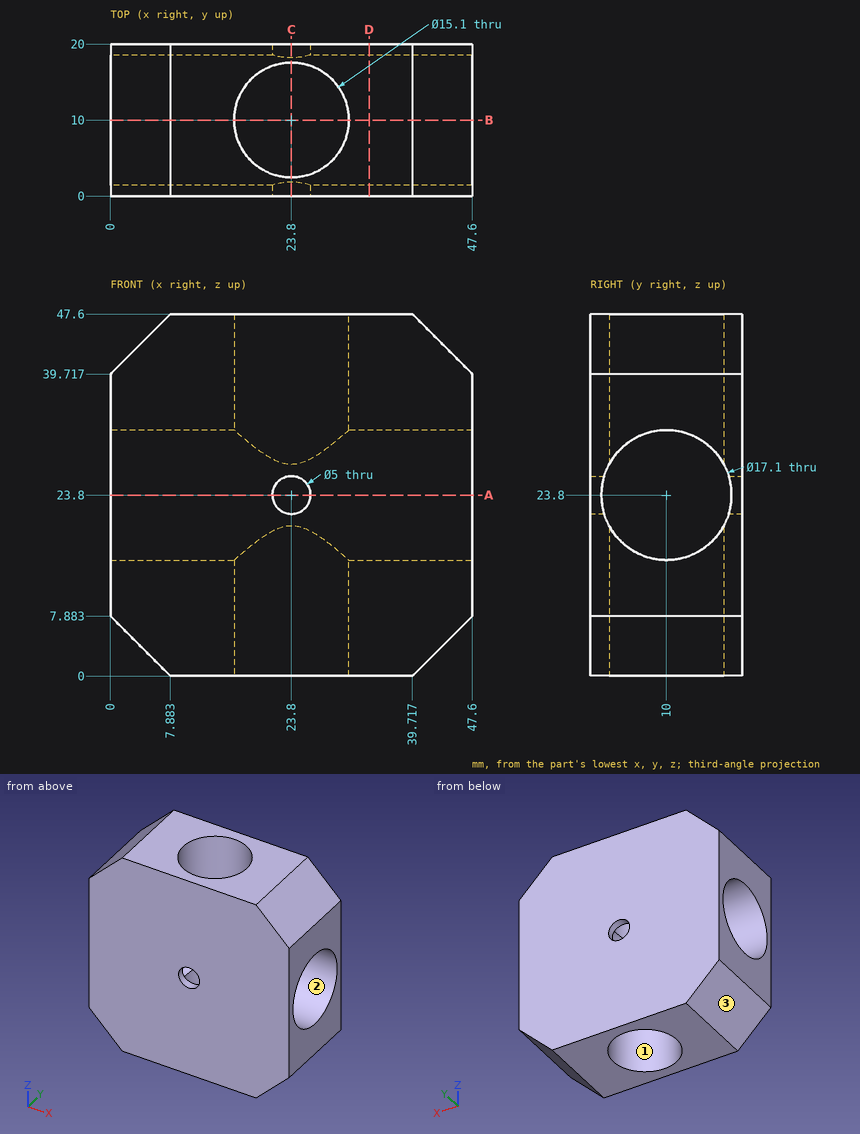
Drawing for the job (mm, zero at the part's lowest x, y, z). Round coordinates to 2 decimals unless told otherwise and drop trailing zeros. Write each loop counter-clockwise with the first axis right and the second up, starting at its lowest first coordinate (ties: lowest second). Pieces come first, ordered by that corner, then holes. Notation, with made-up numbers: M 51,-14 L 108,-14 A34 cw 108,20 Z; hole C -18,27 d10. An arc over 180 degrees is marked long. Answer in a Markdown table with one row per item.
1. Saw through at C-C (x = 23.8). List the corners of the cut face in (y, z).
Geometry check:
| item | result |
|---|---|
| outline | M 0,0 L 2.45,0 L 2.45,19.79 A8.55 cw 1.82,21.3 L 0,21.3 Z; M 0,26.3 L 1.82,26.3 A8.55 cw 2.45,27.81 L 2.45,47.6 L 0,47.6 Z; M 17.55,0 L 20,0 L 20,21.3 L 18.18,21.3 A8.55 cw 17.55,19.79 Z; M 17.55,27.81 A8.55 cw 18.18,26.3 L 20,26.3 L 20,47.6 L 17.55,47.6 Z |
2. Probe L1, parallel to Y at x = 10, z = 24; L2, parallel to X at y = 19.3, z = 23.8; L3, parallel to Y at x = 23.8, z = 7. List the from-to ranges inside material, lowest first. Write a range as [from, to].
Geometry check:
| item | result |
|---|---|
| L1 | [0, 1.45], [18.55, 20] |
| L2 | [0, 21.3], [26.3, 47.6] |
| L3 | [0, 2.45], [17.55, 20] |
3. Mould opens along Z. For the marked faces 1, 2 and 3 say: +Z half, -Z half, draft (parallel to the pull), parting line (faces both ways), or undercut.
Geometry check:
| item | result |
|---|---|
| face 1 | draft |
| face 2 | undercut |
| face 3 | -Z half |
4. Saw through at B-B (y = 10). List the corners of the cut face in (x, z), and give its area (3 significant figures).
Geometry check:
| item | result |
|---|---|
| outline | M 0,7.88 L 7.88,0 L 16.25,0 L 16.25,15.25 L 0,15.25 Z; M 0,32.35 L 16.25,32.35 L 16.25,47.6 L 7.88,47.6 L 0,39.72 Z; M 31.35,0 L 39.72,0 L 47.6,7.88 L 47.6,15.25 L 31.35,15.25 Z; M 31.35,32.35 L 47.6,32.35 L 47.6,39.72 L 39.72,47.6 L 31.35,47.6 Z |
| area | 867 mm2 |
5. Saw through at A-A (z = 23.8). List the corners of the cut face in (x, y).
Geometry check:
| item | result |
|---|---|
| outline | M 0,0 L 21.3,0 L 21.3,1.45 L 0,1.45 Z; M 0,18.55 L 21.3,18.55 L 21.3,20 L 0,20 Z; M 26.3,0 L 47.6,0 L 47.6,1.45 L 26.3,1.45 Z; M 26.3,18.55 L 47.6,18.55 L 47.6,20 L 26.3,20 Z |
6. Saw through at D-D (x = 34). List the corners of the cut face in (y, z), and give its area (3 significant figures).
Geometry check:
| item | result |
|---|---|
| outline | M 0,0 L 20,0 L 20,47.6 L 0,47.6 Z; hole C 10,23.8 d17.1 |
| area | 722 mm2 |
